Source: CAD feature listing. Evaluate the final solid. Frame: model axes, mm. Give positions to 0.01 mm unless a question says otherwise; leave off trailing zeros. Order: outer loops, then holes, each group sorted by start corner. A loop starts at its lowest first (then second) coordinate and runs counter-clockwise, first axis right, second up.
1) Draft query along X for faces 1 (the face through (14, -60.149, 4)), 2 (the face through (23.23, -59.05, 3.79)), 3 (the face through (26.638, -57, 4)). Return one class per face: released by +X, released by -X, zero draft, split by the parting line, or undercut.
2) Section D-D, the plane x = 22.5. Return loops of the section in (y, z).
3) Section C-C, the plane z = 3.25. Return loops of the section in (x, y), plus the area to 3 significant figures.
4) Section A-A, the plane x = 5.75. Return loops of the section in (y, z), plus the area to 3 significant figures.
5) Material intervals for line 1 (X direction, y = -57, z = 3.55); line 2 (X direction, y = -57.5, z = 3.15); line 3 (Y direction, x = 5.25, z = 3.9), sorted ascending.
6) Section B-B, the plane y = -56. Return loops of the section in (x, z), plus the area to 3 significant figures.
```python
from build123d import *

# Parameters (mm, degrees)
ESQUISSE2_W        = 25.4
ESQUISSE2_H        = 6.35
BOSS_EXTRU_1_DEPTH = 1.55
D_GAGEMENT_61_D    = 4.3053


with BuildPart() as part:
    # Esquisse2 → Boss.-Extru.1 (new body)
    with BuildSketch(Plane.XY.offset(3)):
        with Locations((13.938249305, -56.974105441)):
            Rectangle(ESQUISSE2_W, ESQUISSE2_H)
    extrude(amount=BOSS_EXTRU_1_DEPTH)

    # Dégagement #61 (through all)
    with Locations(Plane(origin=(0, 0, 3), x_dir=(-1, 0, 0), z_dir=(0, 0, -1))):
        with Locations((-4.138249305, -56.949105441), (-23.698249305, -56.949105441)):
            Hole(D_GAGEMENT_61_D / 2)


solid = part.part
```
From the geometry:
1. face 1: zero draft
1. face 2: undercut
1. face 3: released by +X
2. outline: (-60.15, 3) - (-58.74, 3) - (-58.74, 4.55) - (-60.15, 4.55) - close; (-55.16, 3) - (-53.8, 3) - (-53.8, 4.55) - (-55.16, 4.55) - close
3. outline: (1.24, -60.15) - (26.64, -60.15) - (26.64, -53.8) - (1.24, -53.8) - close; hole circle Ø4.31 at (4.14, -56.95); hole circle Ø4.31 at (23.7, -56.95)
3. area: 132 mm2
4. outline: (-60.15, 3) - (-58.38, 3) - (-58.38, 4.55) - (-60.15, 4.55) - close; (-55.52, 3) - (-53.8, 3) - (-53.8, 4.55) - (-55.52, 4.55) - close
4. area: 5.42 mm2
5. line 1: x = 1.24 to 1.99, 6.29 to 21.55, 25.85 to 26.64
5. line 2: x = 1.24 to 2.06, 6.22 to 21.62, 25.78 to 26.64
5. line 3: y = -60.15 to -58.79, -55.11 to -53.8
6. outline: (1.24, 3) - (2.21, 3) - (2.21, 4.55) - (1.24, 4.55) - close; (6.07, 3) - (21.77, 3) - (21.77, 4.55) - (6.07, 4.55) - close; (25.63, 3) - (26.64, 3) - (26.64, 4.55) - (25.63, 4.55) - close
6. area: 27.4 mm2
